Verification items for the finished model (mm, model axes). Round coordinates to 2 decimals unless told otherwise and drop trailing zeros. Order: outer loops, then holes, each group sorted by start corner. A loop starts at its lowest first (then second) coordinate and runs counter-clockwise, first axis right, second up. Notation, with made-up numbers: M 61,-10.75 L 89,-10.75 A26 cw 89,25.25 Z; hole C 72.25,-15 d10. An arc over 180 degrees is marked long. Write item = value, one per line. Start each with the question number.
from build123d import *

# Parameters (mm, degrees)
SKETCH1_W           = 121
SKETCH1_H           = 85
BOSS_EXTRUDE1_DEPTH = 2
SKETCH4_W           = 101
SKETCH4_H           = 65
CUT_EXTRUDE1_DEPTH  = 148.885090526
SKETCH5_R           = 1.5
CUT_EXTRUDE2_DEPTH  = 148.885090526


with BuildPart() as part:
    # Sketch1 → Boss-Extrude1 (new body)
    with BuildSketch(Plane.XY):
        with Locations((60.5, 42.5)):
            Rectangle(SKETCH1_W, SKETCH1_H)
    extrude(amount=BOSS_EXTRUDE1_DEPTH)

    # Sketch4 → Cut-Extrude1 (cut, through all)
    with BuildSketch(Plane.XY.offset(2)):
        with Locations((60.5, 42.5)):
            Rectangle(SKETCH4_W, SKETCH4_H)
    extrude(amount=-CUT_EXTRUDE1_DEPTH, mode=Mode.SUBTRACT)

    # Sketch5 → Cut-Extrude2 (cut, through all)
    with BuildSketch(Plane.XY.offset(2)):
        with Locations((6, 79)):
            Circle(SKETCH5_R)
        with Locations((115, 79)):
            Circle(SKETCH5_R)
        with Locations((6, 6)):
            Circle(SKETCH5_R)
        with Locations((115, 6)):
            Circle(SKETCH5_R)
    extrude(amount=-CUT_EXTRUDE2_DEPTH, mode=Mode.SUBTRACT)


solid = part.part
1) Cross-section at B-B, the plane y = 79. Enter the section's corners in (x, z).
2) Cross-section at A-A, the plane x = 115. Enter the section's corners in (y, z), then the cut area to 3 significant figures.
3) Scan lines: probe 1 along Y at (x, z) = (115, 0.5); probe 2 along Y at (x, z) = (21, 1.45); probe 3 along X at (y, z) = (12, 1.2). Record each from-to range of solid material in increasing order.
4) Gauge pin test, flat ends, axial feed: P1, Ø12, axis at x = 57, y = 68.5, coming from the -Z side; P2, Ø4, axis at x = 115, y = 79, coming from the +Z side. Record the tip position at first contact, or that the pin passes through.
5) Release check for a two-part mould opening along X. For faces 1 (the cylindrical face through (5.805, 80.487, 1.014)), 2 (the flat face through (60, 81, 0)) record: pulls with the +X half, pulls with the -X half, needs draft (parallel to the pull), parting line crosses it, or undercut.
6) Cross-section at C-C, the plane y = 22. Enter the section's corners in (x, z).
7) Cross-section at D-D, the plane z = 0.7. Enter the section's corners in (x, y), then the cut area to 3 significant figures.
Geometry results:
q1.outline = M 0,0 L 4.5,0 L 4.5,2 L 0,2 Z; M 7.5,0 L 113.5,0 L 113.5,2 L 7.5,2 Z; M 116.5,0 L 121,0 L 121,2 L 116.5,2 Z
q2.outline = M 0,0 L 4.5,0 L 4.5,2 L 0,2 Z; M 7.5,0 L 77.5,0 L 77.5,2 L 7.5,2 Z; M 80.5,0 L 85,0 L 85,2 L 80.5,2 Z
q2.area = 158 mm^2
q3.probe_1 = 0 to 4.5, 7.5 to 77.5, 80.5 to 85
q3.probe_2 = 0 to 10, 75 to 85
q3.probe_3 = 0 to 10, 111 to 121
q4.P1 = through
q4.P2 = 2
q5.face_1 = undercut
q5.face_2 = needs draft
q6.outline = M 0,0 L 10,0 L 10,2 L 0,2 Z; M 111,0 L 121,0 L 121,2 L 111,2 Z
q7.outline = M 0,0 L 121,0 L 121,85 L 0,85 Z; hole C 6,6 d3; hole C 6,79 d3; hole M 10,10 L 111,10 L 111,75 L 10,75 Z; hole C 115,6 d3; hole C 115,79 d3
q7.area = 3,690 mm^2
